Design review of the part built by this model. Coordinates are the model's own, in mm. A direction names the side the tool comes from. Coordinates: 2 decimals unless noted, no trailing zeros. Loops run counter-clockwise (first coordinate to the right, second up) from the corner with the lowest first, then second, coordinate; pieces in that order, holes last. Notation, with made-up numbers: M 68.25,50.5 L 84.25,50.5 A22 cw 84.25,65.5 Z; hole C -29,40 d10. An arc over 180 degrees is marked long. Put each result on its own line as item: value. Start each with the question number.
(1) Take a section at A-A, the plane y = 0. Give the boundary of the cut face in (x, z).
(2) Take a section at D-D, the plane z = 0.75. Give the boundary of the cut face in (x, y), then the cut area to 3 significant figures.
(3) Take a section at C-C, the plane z = 4.75. Give the boundary of the cut face in (x, y).
(4) For faces 1 (the cylindrical face through (-0.27, -1.22, 4.98)), 2 (the cylindrical face through (-0.27, -1.22, -4.98)), 3 (the cylindrical face through (0.715, -1.375, 0.053)), list the 3-axis set-ups (+Z, -Z, +X, -X, +Y, -Y) from which the entire face can be reached by the end or side of a thin tool; tool diameter is ignored.
(5) For probe 1 along Z at (x, y) = (-1.3, -0.55); probe 2 along Y at (x, z) = (0.1, 3.25); probe 3 along X at (y, z) = (-0.9, 3.5), list the stretches that pass through material, from the lowest coordinate up. Write a range as [from, to].
(6) Take a section at B-B, the plane x = -0.2. Give the boundary of the cut face in (y, z), then the cut area to 3 significant figures.
```python
from build123d import *

# Parameters (mm, degrees)
SKETCH2_R           = 1.55
BOSS_EXTRUDE2_DEPTH = 3.75
SKETCH4_R           = 1.25
BOSS_EXTRUDE3_DEPTH = 2.5


with BuildPart() as part:
    # Sketch2 → Boss-Extrude2 (new body)
    with BuildSketch(Plane.XY):
        Circle(SKETCH2_R)
    boss_extrude2 = extrude(amount=BOSS_EXTRUDE2_DEPTH)

    # Sketch4 → Boss-Extrude3 (add)
    with BuildSketch(Plane.XY.offset(3.75)):
        Circle(SKETCH4_R)
    boss_extrude3 = extrude(amount=BOSS_EXTRUDE3_DEPTH)

    # Mirror3: Boss-Extrude2, Boss-Extrude3 across plane
    add(boss_extrude2.mirror(Plane.XY))
    add(boss_extrude3.mirror(Plane.XY))


solid = part.part
```
Computed values:
1. outline: M -1.55,-3.75 L -1.25,-3.75 L -1.25,-6.25 L 1.25,-6.25 L 1.25,-3.75 L 1.55,-3.75 L 1.55,3.75 L 1.25,3.75 L 1.25,6.25 L -1.25,6.25 L -1.25,3.75 L -1.55,3.75 Z
2. outline: C 0,0 d3.1
2. area: 7.55 mm^2
3. outline: C 0,0 d2.5
4. face 1: +Z
4. face 2: -Z
4. face 3: +Z, -Z
5. probe 1: z = [-3.75, 3.75]
5. probe 2: y = [-1.55, 1.55]
5. probe 3: x = [-1.26, 1.26]
6. outline: M -1.54,-3.75 L -1.23,-3.75 L -1.23,-6.25 L 1.23,-6.25 L 1.23,-3.75 L 1.54,-3.75 L 1.54,3.75 L 1.23,3.75 L 1.23,6.25 L -1.23,6.25 L -1.23,3.75 L -1.54,3.75 Z
6. area: 35.4 mm^2
